Input: part model. Units: mm. Frame: model coordinates. Face numbers are marked on the shaded views. A direction names the side the tool comes from. Coordinates: 2 decimals unless noted, no trailing zeros. Loops run counter-clockwise (first coordinate to the right, second up) from the corner with the lowest first, then second, coordinate; pieces in that order, holes last. Notation, with made-up numbers: (-8, 6) - (37, 6) arc R9 cw to (37, 13) - close; hole circle Ø4 at (63, -16.5). An arc over 180 degrees is marked (long way). Use one line per item in the form item = value.
from build123d import *

# Parameters (mm, degrees)
F1_DEPTH = 25.4
F2_W     = 16.371028
F2_H     = 25.4
F3_DEPTH = 25.4
F4_R     = 1.905
F5_DEPTH = 25.4


with BuildPart() as f1:
    # F0 (on Front) → F1 (new body)
    with BuildSketch(Plane.XZ):
        Polygon((-18.553972, 20.450408), (-21.728972, 20.450408), (-21.728972, -17.649592), (16.371028, -17.649592), (16.371028, -14.474592), (-18.553972, -14.474592), align=None)
    extrude(amount=F1_DEPTH)

    # F2 (on face) → F3 (cut)
    with BuildSketch(Plane(origin=(0, 0, -17.649592), x_dir=(1, 0, 0), z_dir=(0, 0, -1))):
        with Locations((8.185514, 12.7)):
            Rectangle(F2_W, F2_H)
    extrude(amount=-F3_DEPTH, mode=Mode.SUBTRACT)

    # F4 (on face) → F5 (cut)
    with BuildSketch(Plane(origin=(-21.728972, 0, 0), x_dir=(0, -1, 0), z_dir=(-1, 0, 0))):
        with Locations((12.7, 4.702408)):
            Circle(F4_R)
    extrude(amount=-F5_DEPTH, mode=Mode.SUBTRACT)


solid = f1.part
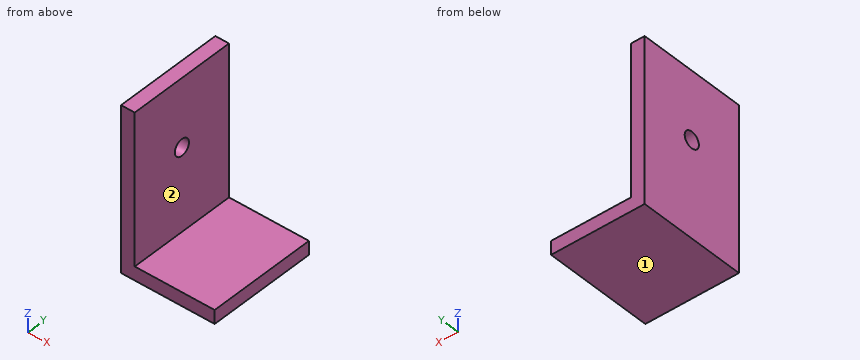
Q1. Ray query, line 1 along Z through (x, y) = (-21, -12.7); line 2 along X through (y, z) = (-12.25, -11); line 3 along Z through (x, y) = (-19.5, -11.75). Return the intervals inside material, ascending. Write a range as [from, to].
Check values:
line_1 = [-17.65, 2.8], [6.61, 20.45]
line_2 = [-21.73, -18.55]
line_3 = [-17.65, 3.05], [6.35, 20.45]
Q2. Cut plane C-C, the plane z = 14.5. Return loops of the section in (x, y), then the cut area to 3 significant figures.
Check values:
outline = (-21.73, -25.4) - (-18.55, -25.4) - (-18.55, 0) - (-21.73, 0) - close
area = 80.6 mm²
Q3. Cut plane B-B, the plane y = -23. Return loops of the section in (x, z).
Check values:
outline = (-21.73, -17.65) - (0, -17.65) - (0, -14.47) - (-18.55, -14.47) - (-18.55, 20.45) - (-21.73, 20.45) - close
Q4. Cut plane D-D, the plane x = -15. Return loops of the section in (y, z).
Check values:
outline = (-25.4, -17.65) - (0, -17.65) - (0, -14.47) - (-25.4, -14.47) - close
Q5. Set-up query: the marked faces 1 and 2. Return all of +Z, -Z, +X, -X, +Y, -Y with unobstructed straight access to the full face (end or side cutting, diameter ignored); none if empty.
Check values:
face_1 = -Z, +X, -X, +Y, -Y
face_2 = +Z, +X, +Y, -Y
Q6. First-contact query: P1, Ø4, axis at y = -10, z = 6, coming from the +X side; P2, Ø2.5, axis at y = -12.7, z = 4.7, coming from the +X side; P3, Ø5.5, axis at x = -12, y = -17, coming from the +Z side. Flat tips, straight axial feed; report the tip coordinate or a pass-through.
Check values:
P1 = -18.55
P2 = through
P3 = -14.47
Q7. Cut plane A-A, the plane y = -12.7. Return loops of the section in (x, z), then the cut area to 3 significant figures.
Check values:
outline = (-21.73, -17.65) - (0, -17.65) - (0, -14.47) - (-18.55, -14.47) - (-18.55, 2.8) - (-21.73, 2.8) - close; (-21.73, 6.61) - (-18.55, 6.61) - (-18.55, 20.45) - (-21.73, 20.45) - close
area = 168 mm²
